The figure shows three views and two pictorial views of one solid part (mm, origin at its lowest corner). Answer the questions. A direction names the side the tool comes from. Round coordinates to 2 decimals unless told otherwise and drop trailing zeros. Order: outer loops, then holes, each group sorted by start corner. A loop starts at its lowest first (then second) coordinate and runs counter-clockwise, first axis right, second up. Notation, with made-up numbers: (60.5, 24) - (110.5, 24) arc R7 cw to (110.5, 32) - close; hole circle Ø1 at (8, 84). An arc over 180 degrees is marked (long way). Answer in a Markdown table with one row per item.
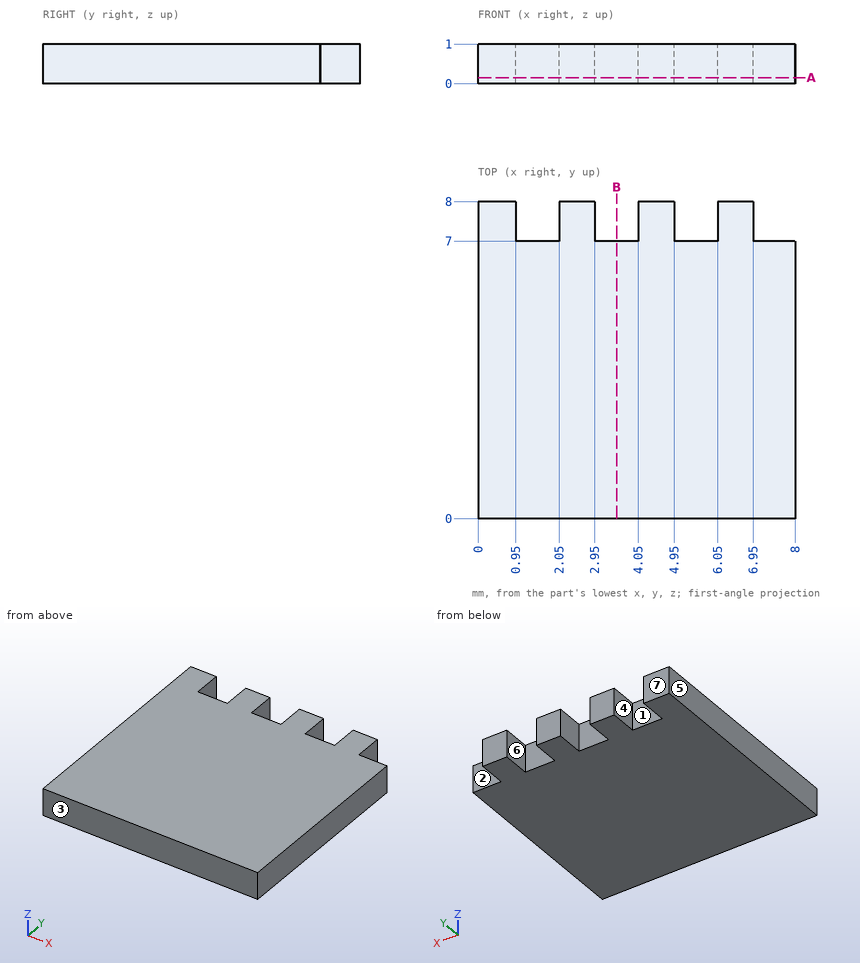
1) Which of the six approach directions +Z, -Z, +X, -X, +Y, -Y give full straight-line access (tool end or side, diameter ignored) to the marked faces 1, 2 and 3?
Filled in:
| item | result |
|---|---|
| face 1 | +Z, -Z, +Y |
| face 2 | +Z, -Z, +X, +Y |
| face 3 | +Z, -Z, +X, -X, -Y |
2) Find the intervals of material crossed by probe 1 along Y at (x, z) = (5.5, 0.9), in increasing order. Write a range as from..to.
Filled in:
| item | result |
|---|---|
| probe 1 | y = 0..7 |
3) The mould has two halves that part along X. Classify the marked faces 4, 5, 6 and 7: released by +X, released by -X, zero draft, split by the parting line, or undercut.
Filled in:
| item | result |
|---|---|
| face 4 | undercut |
| face 5 | released by -X |
| face 6 | undercut |
| face 7 | zero draft |
4) Find section A-A, the plane z = 0.15. Give the vertices of the cut face in (x, y), then the cut area to 4 significant figures.
Filled in:
| item | result |
|---|---|
| outline | (0, 0) - (8, 0) - (8, 7) - (6.95, 7) - (6.95, 8) - (6.05, 8) - (6.05, 7) - (4.95, 7) - (4.95, 8) - (4.05, 8) - (4.05, 7) - (2.95, 7) - (2.95, 8) - (2.05, 8) - (2.05, 7) - (0.95, 7) - (0.95, 8) - (0, 8) - close |
| area | 59.65 mm^2 |
5) Each of these flat-tipped pins is pushed along its axis until it touches: pin 1 (0.5 mm diameter, centred on y = 7.5, z = 0.5, fed in from +X); pin 2 (0.5 mm diameter, centred on x = 5.5, z = 0.5, fed in from +Y). Where does it stop, or does it pass through?
Filled in:
| item | result |
|---|---|
| pin 1 | stops at x = 6.95 |
| pin 2 | stops at y = 7 |
6) Find section B-B, the plane x = 3.5. Give the vertices of the cut face in (y, z).
Filled in:
| item | result |
|---|---|
| outline | (0, 0) - (7, 0) - (7, 1) - (0, 1) - close |
